The drawing under review shows one solid part. Ordinate dimensions are in mm from its lowest x, y, z. A direction names the side the tool comes from. Give positions to 0.01 mm unless a question says otherwise; leave off trailing zeros. Order: outer loops, then holes, each group sorted by start corner. A loop starts at its lowest first (then second) coordinate and runs counter-clockwise, first axis right, second up. Notation, with made-up numbers: (-23.5, 4.25) -> (17.5, 4.25) arc R26 ccw to (17.5, 24.25) -> close; hole circle Ø11 at (61.5, -26.5). An arc over 180 degrees is marked (long way). Use a Markdown table: item, result. Add a question column.
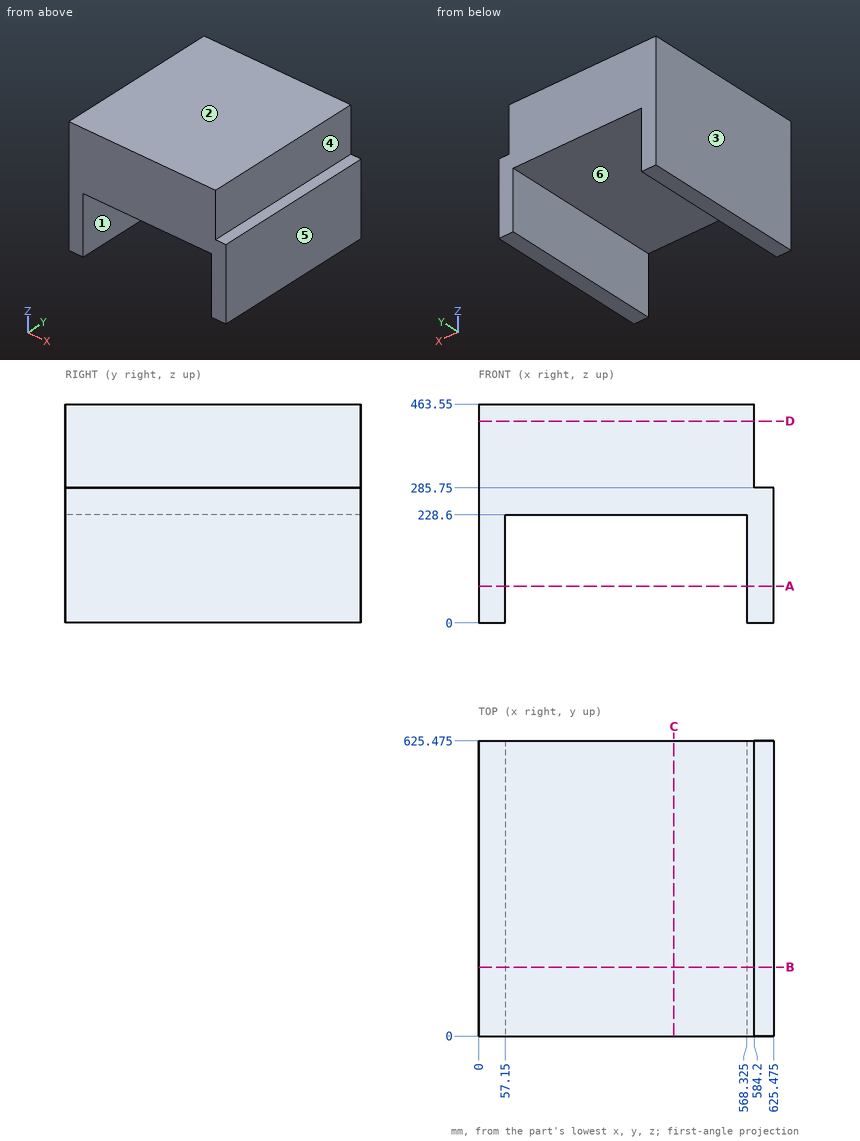
1) The part is to be moulded in two halves that separate along X. For the marked faces 1, 2, 3 and 4, say which applies: +X half, -X half, draft (parallel to the pull), parting line (faces both ways), or undercut.
2) Add section B-B (y = 146). Give the boundary of the cut face in (x, z) (3 decimals).
3) Machinability: for the marked faces 5 and 6, which of the approach directions +Z, -Z, +X, -X, +Y, -Y give a long, thin tool a straight path to every point of the face, cutting with its end or side? Answer none if there is none.
4) Insertion check: pin 1 (10 mm diameter, centred on x = 558.5, z = 150.5, fed in from -Y); pin 2 (3 mm diameter, centred on x = 89.5, y = 423.5, fed in from -Z); pin 3 (10 mm diameter, centred on y = 212, z = 298.5, fed in from +X). Each pin has a flat end and moves straight along its axis. Give the tip position at first contact, or say it passes through.
5) Add section A-A (z = 77.5). Give the boundary of the cut face in (x, y) (3 decimals).
6) For L1, parallel to X at y = 337, z = 81 (3 decimals); L2, parallel to Z at x = 350, y = 45; L3, parallel to X at y = 239, z = 433.5, list the stretches that pass through material, from the lowest coordinate up. Write a range as [from, to].
7) Add section C-C (x = 414). Give the boundary of the cut face in (y, z) (3 decimals), then the cut area to 3 significant figures.
8) Add section D-D (z = 427). Give the boundary of the cut face in (x, y) (3 decimals).
Worked answers:
| question | item | result |
|---|---|---|
| 1 | face 1 | undercut |
| 1 | face 2 | draft |
| 1 | face 3 | -X half |
| 1 | face 4 | +X half |
| 2 | outline | (0, 0) -> (57.15, 0) -> (57.15, 228.6) -> (568.325, 228.6) -> (568.325, 0) -> (625.475, 0) -> (625.475, 285.75) -> (584.2, 285.75) -> (584.2, 463.55) -> (0, 463.55) -> close |
| 3 | face 5 | +Z, -Z, +X, +Y, -Y |
| 3 | face 6 | -Z, +Y, -Y |
| 4 | pin 1 | through |
| 4 | pin 2 | z = 228.6 |
| 4 | pin 3 | x = 584.2 |
| 5 | outline | (0, 0) -> (57.15, 0) -> (57.15, 625.475) -> (0, 625.475) -> close; (568.325, 0) -> (625.475, 0) -> (625.475, 625.475) -> (568.325, 625.475) -> close |
| 6 | L1 | [0, 57.15], [568.325, 625.475] |
| 6 | L2 | [228.6, 463.55] |
| 6 | L3 | [0, 584.2] |
| 7 | outline | (0, 228.6) -> (625.475, 228.6) -> (625.475, 463.55) -> (0, 463.55) -> close |
| 7 | area | 147,000 mm^2 |
| 8 | outline | (0, 0) -> (584.2, 0) -> (584.2, 625.475) -> (0, 625.475) -> close |
